Work out the finished part from the listing and answer in its coordinate system (mm). A direction names the side the tool comes from. Coordinates: 2 decimals unless noted, no trailing zeros. Write each loop counter-clockwise with the first axis right and the second up, starting at its lowest first coordinate (ties: lowest second). Pieces come first, ordered by that corner, then holes. Notation, with made-up numbers: (65.5, -38.5) - (114.5, -38.5) arc R22 cw to (114.5, -14.5) - close; hole circle Ø10 at (88.5, 36). An arc over 180 degrees is marked (long way). Use a Markdown table: item, result. Add a question column.
(1) For a pull along Z with two mould halves and no side action, classify faces 1 (the face through (40.355, 6.965, -0.499)), 2 (the face through (21, 22.9, 9)), 3 (the face through (21.1, 5.8, 11)) as released by +Z, released by -Z, zero draft, split by the parting line, or undercut.
(2) Given pin 1 Ø7 at (x, z) = (-1, 1) entering from +Y; pin 2 Ø0.5 at (x, y) = (0.5, 7) entering from -Z; pin 3 Ø6 at (x, y) = (40.5, 10) entering from -Z; pin 4 Ø5 at (x, y) = (23, 17) entering from +Z, each flat-ended and moving along its own axis, determine where each tip first touches the part or whether it passes through.
(3) The part is cut by section B-B, the plane y = 8. Give the vertices of the cut face in (x, z).
(4) The part is cut by section A-A, the plane z = 0. Give the vertices of the cut face in (x, y).
(5) The part is cut by section C-C, the plane x = 19.5. Give the vertices of the cut face in (y, z), then the cut area to 3 significant figures.
(6) Find the intervals of material crossed by line 1 (X direction, y = 5.65, z = 0); line 2 (X direction, y = 9.25, z = -1); line 3 (Z direction, x = 42.6, y = 5.8), in increasing order. Write a range as from..to.
(7) The part is cut by section D-D, the plane y = 12. Give the vertices of the cut face in (x, z).
(8) A tool of negligible diameter and unlimited length cuts with its end or side. For faces 4 (the face through (3, 9.5, -1)), 5 (the face through (49.59, 6.96, -0.36)), 6 (the face through (21, 6.1, 9)), 7 (the face through (42, 7, -7)), 8 (the face through (35.6, 12, -1)), from which of +Z, -Z, +X, -X, +Y, -Y can it reach the whole face along a straight path? Write none if from no direction.
from build123d import *

# Parameters (mm, degrees)
SKETCH1_R                = 2.3
BOSS_EXTRUDE1_DEPTH      = 9.5
BOSS_EXTRUDE2_DEPTH      = 15
BOSS_EXTRUDE2_DEPTH_BACK = 9.5
SKETCH2_W                = 28.6
SKETCH2_H                = 19.5
SKETCH3_R                = 7.5
CUT_EXTRUDE1_DEPTH       = 59.657139378
FILLET1_R                = 10
FILLET2_R                = 6
CUT_EXTRUDE2_REACH       = 60.657
SKETCH5_W                = 56.6
SKETCH5_H                = 4.5
BOSS_EXTRUDE3_DEPTH      = 4
FILLET3_R                = 10


with BuildPart() as part:
    # Sketch1 → Boss-Extrude1 (new body)
    with BuildSketch(Plane(origin=(0, 0, 0), x_dir=(1, 0, 0), z_dir=(0, 1, 0))):
        with BuildLine():
            Line((0, 7), (42.6, 7))
            ThreePointArc((42.6, 7), (49.6, 0), (42.6, -7))
            Line((42.6, -7), (0, -7))
            ThreePointArc((0, -7), (-7, 0), (0, 7))
        make_face()
        with Locations(Location((0, 0, 0), (0, 0, 270))):
            Circle(SKETCH1_R, mode=Mode.SUBTRACT)
        with Locations(Location((42.6, 0, 0), (0, 0, 270))):
            Circle(SKETCH1_R, mode=Mode.SUBTRACT)
    extrude(amount=BOSS_EXTRUDE1_DEPTH)

    # Sketch2 → Boss-Extrude2 (add, two sides: drawn at the far end of the back side and taken through both)
    with BuildSketch(Plane(origin=(0, 9.5, 0), x_dir=(1, 0, 0), z_dir=(0, 1, 0)).offset(-BOSS_EXTRUDE2_DEPTH_BACK)):
        with Locations((21.3, 2.75)):
            Rectangle(SKETCH2_W, SKETCH2_H)
    extrude(amount=BOSS_EXTRUDE2_DEPTH + BOSS_EXTRUDE2_DEPTH_BACK)

    # Sketch3 → Cut-Extrude1 (cut, through all)
    with BuildSketch(Plane(origin=(0, 0, -12.5), x_dir=(-1, 0, 0), z_dir=(0, 0, -1))):
        with Locations((-21.3, 14.5)):
            Circle(SKETCH3_R)
    extrude(amount=-CUT_EXTRUDE1_DEPTH, mode=Mode.SUBTRACT)

    # Fillet1
    fillet1_edges = [part.edges().sort_by_distance(p)[0] for p in [
        (7, 24.5, -2.75),
        (35.6, 24.5, -2.75),
    ]]
    fillet(fillet1_edges, radius=FILLET1_R)

    # Fillet2
    # the kernel refuses this fillet: 6 mm, written as the material it adds along each edge
    with BuildSketch(Plane(origin=(7, 0, -7), x_dir=(0, 0, -1), z_dir=(0, 1, 0)), Plane(origin=(35.6, 9.5, -7), x_dir=(0, 0, -1), z_dir=(0, -1, 0))) as fillet2_piece_1:
        with BuildLine():
            CenterArc((6, 5.979130372), FILLET2_R, 180, 85.219808153)
            Line((0, 5.979130372), (-0.12, 5.979130372))
            Line((-0.12, 5.979130372), (-0.12, 0))
            Line((-0.12, 0), (0, -0.12))
            ThreePointArc((0, -0.12), (2.75, -0.12), (5.49, -0.119582607))
            Line((5.49, -0.119582607), (5.5, 0))
        make_face()
    extrude(amount=9.5)

    # Sketch5 → Cut-Extrude2 (cut, up to next)
    with BuildSketch(Plane(origin=(0, 0, -12.5), x_dir=(-1, 0, 0), z_dir=(0, 0, -1)), mode=Mode.PRIVATE) as cut_extrude2_sk1:
        with Locations((-21.3, 2.25)):
            Rectangle(SKETCH5_W, SKETCH5_H)
    cut_extrude2_tool1 = extrude(cut_extrude2_sk1.sketch, amount=-CUT_EXTRUDE2_REACH, mode=Mode.PRIVATE) & part.part
    add(cut_extrude2_tool1.solids().sort_by_distance((21.3, 2.25, -12.5))[0], mode=Mode.SUBTRACT)

    # Sketch10 → Boss-Extrude3 (add)
    with BuildSketch(Plane(origin=(0, 0, 7), x_dir=(-1, 0, 0), z_dir=(0, 0, -1))):
        with BuildLine():
            Line((-35.6, 4.5), (-35.6, 14.5))
            ThreePointArc((-35.6, 14.5), (-32.671067812, 21.571067812), (-25.6, 24.5))
            Line((-25.6, 24.5), (-17, 24.5))
            ThreePointArc((-17, 24.5), (-9.928932188, 21.571067812), (-7, 14.5))
            Line((-7, 14.5), (-7, 4.5))
            Line((-7, 4.5), (-35.6, 4.5))
        make_face()
        Polygon((-16.450257739, 22.9), (-26.149742261, 22.9), (-30.999484522, 14.5), (-26.149742261, 6.1), (-16.450257739, 6.1), (-11.600515478, 14.5), align=None, mode=Mode.SUBTRACT)
    extrude(amount=-BOSS_EXTRUDE3_DEPTH)

    # Fillet3
    # the kernel refuses this fillet: 10 mm, written as the material it adds along each edge
    with BuildSketch(Plane(origin=(7, 9.5, 7), x_dir=(-0.9999985389310836, 0, -0.0017094255462351089), z_dir=(0, -1, 0))) as fillet3_piece_1:
        with BuildLine():
            CenterArc((8.005961044, -9.982891134), FILLET3_R, 93.352047646, 49.900448128)
            Line((-0.006837702, -3.999994156), (-0.808117577, -3.401704458))
            ThreePointArc((-0.808117577, -3.401704458), (-1.00341739, -1.998287652), (-0.999998539, 0.001709426))
            Line((-0.999998539, 0.001709426), (0.001709426, 0.999998539))
            ThreePointArc((0.001709426, 0.999998539), (7.001699198, 0.98803256), (7.362781149, 0.998289113))
            Line((7.362781149, 0.998289113), (7.421252048, 0))
        make_face()
    extrude(amount=5)
    with BuildSketch(Plane(origin=(35.6, 4.5, 7), x_dir=(0, 0, 1), z_dir=(0, 1, 0))) as fillet3_piece_2:
        with BuildLine():
            CenterArc((9.969190954, 8.023014356), FILLET3_R, 183.449990563, 49.900448128)
            Line((-0.012686078, 7.421241205), (-1.010873781, 7.36106389))
            ThreePointArc((-1.010873781, 7.36106389), (-1, 7), (-1, 0))
            Line((-1, 0), (0, -1))
            ThreePointArc((0, -1), (2, -1), (3.403080905, -0.802301436))
            Line((3.403080905, -0.802301436), (4, 0))
        make_face()
    extrude(amount=5)


solid = part.part
Model answer:
| question | item | result |
|---|---|---|
| 1 | face 1 | undercut |
| 1 | face 2 | zero draft |
| 1 | face 3 | released by +Z |
| 2 | pin 1 | y = 9.5 |
| 2 | pin 2 | z = -7 |
| 2 | pin 3 | z = -8.56 |
| 2 | pin 4 | through |
| 3 | outline | (-0.42, 6.99) arc R7 ccw to (0, -7) - (1.02, -7) arc R6 cw to (7, -12.5) - (17.56, -12.5) - (17.56, 7) - (15.35, 7) - (15.35, 11) - (7, 11) arc R10 cw to start; (25.04, -12.5) - (35.6, -12.5) arc R6 cw to (41.58, -7) - (42.6, -7) arc R7 ccw to (43.02, 6.99) arc R10 cw to (35.6, 11) - (27.25, 11) - (27.25, 7) - (25.04, 7) - close; hole circle Ø4.6 at (0, 0); hole circle Ø4.6 at (42.6, 0) |
| 4 | outline | (-7, 4.5) - (-2.3, 4.5) - (-2.3, 9.5) - (-7, 9.5) - close; (2.3, 4.5) - (40.3, 4.5) - (40.3, 9.5) - (35.6, 9.5) - (35.6, 14.5) arc R10 ccw to (25.6, 24.5) - (17, 24.5) arc R10 ccw to (7, 14.5) - (7, 9.5) - (2.3, 9.5) - close; (44.9, 4.5) - (49.6, 4.5) - (49.6, 9.5) - (44.9, 9.5) - close; hole circle Ø15 at (21.3, 14.5) |
| 5 | outline | (4.5, -12.5) - (7.22, -12.5) - (7.22, 7) - (6.1, 7) - (6.1, 11) - (4.5, 11) - close; (21.78, -12.5) - (24.5, -12.5) - (24.5, 11) - (22.9, 11) - (22.9, 7) - (21.78, 7) - close |
| 5 | area | 119 mm^2 |
| 6 | line 1 | -7..-2.3, 2.3..40.3, 44.9..49.6 |
| 6 | line 2 | -6.93..-2.07, 2.07..15.94, 26.66..40.53, 44.67..49.53 |
| 6 | line 3 | -7..-2.3, 2.3..7.02 |
| 7 | outline | (7, -12.5) - (14.23, -12.5) - (14.23, 7) - (13.04, 7) - (13.04, 11) - (7, 11) - close; (28.37, -12.5) - (35.6, -12.5) - (35.6, 11) - (29.56, 11) - (29.56, 7) - (28.37, 7) - close |
| 8 | face 4 | +Z, -Z, -X, +Y |
| 8 | face 5 | +X, +Y, -Y |
| 8 | face 6 | +Z |
| 8 | face 7 | -Z, +X, +Y, -Y |
| 8 | face 8 | +Z, -Z, +X, +Y |
